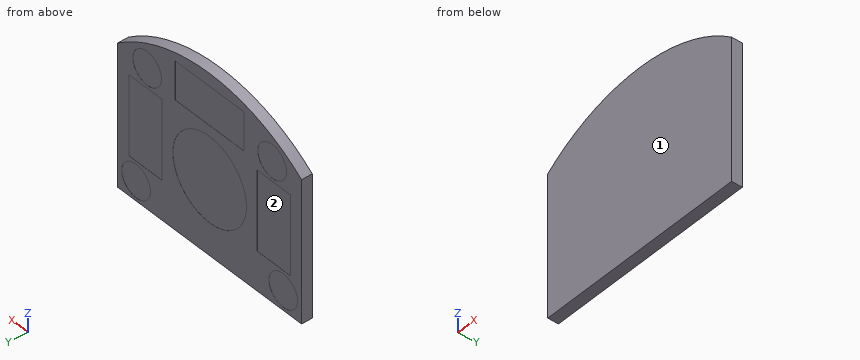
from build123d import *

# Parameters (mm, degrees)
BOSS_EXTRUDE1_DEPTH  = 12.7
BOSS_EXTRUDE2_DEPTH  = 11.176
BOSS_EXTRUDE10_DEPTH = 3.175
SKETCH22_W           = 92.185700808
SKETCH22_H           = 89.424577416
CUT_EXTRUDE13_DEPTH  = 26.4
SKETCH26_W           = 63.5
SKETCH26_H           = 12.7
BOSS_EXTRUDE11_DEPTH = 3.175
SKETCH23_R           = 4.953
SKETCH23_R_2         = 12.7
CUT_EXTRUDE14_DEPTH  = 0.0254
SKETCH25_W           = 11.509375
SKETCH25_H           = 23.8125
SKETCH25_W_2         = 23.8125
SKETCH25_H_2         = 11.509375
CUT_EXTRUDE15_DEPTH  = 0.0254
SKETCH27_W           = 63.5
SKETCH27_H           = 12.7
CUT_EXTRUDE16_DEPTH  = 4.175


with BuildPart() as part:
    # Sketch1 → Boss-Extrude1 (new body)
    with BuildSketch(Plane(origin=(0, 0, 0), x_dir=(1, 0, 0), z_dir=(0, 1, 0))):
        with BuildLine():
            Line((-31.75, 0), (31.75, 0))
            Line((31.75, 0), (31.75, -42.418))
            ThreePointArc((31.75, -42.418), (0, -53.56226271), (-31.75, -42.418))
            Line((-31.75, -42.418), (-31.75, 0))
        make_face()
    extrude(amount=BOSS_EXTRUDE1_DEPTH)

    # Sketch2 → Boss-Extrude2 (add)
    with BuildSketch(Plane.ZY.offset(19.558)):
        with BuildLine():
            Line((0, 0), (-12.7, 0))
            ThreePointArc((-12.7, 0), (-21.680256121, 21.680256121), (0, 12.7))
            Line((0, 12.7), (0, 0))
        make_face()
    boss_extrude2 = extrude(amount=-BOSS_EXTRUDE2_DEPTH)

    # Mirror1: Boss-Extrude2 across plane
    add(boss_extrude2.mirror(Plane(origin=(0, 0, 0), x_dir=(0, 0, 1), z_dir=(1, 0, 0))))

    # Sketch20 → Boss-Extrude10 (add)
    with BuildSketch(Plane.XZ):
        with BuildLine():
            Line((-31.75, 42.418), (-31.75, 0))
            Line((-31.75, 0), (-19.558, 0))
            Line((-19.558, 0), (-19.558, -12.7))
            Line((-19.558, -12.7), (-8.382, -12.7))
            Line((-8.382, -12.7), (-8.382, 0))
            Line((-8.382, 0), (8.382, 0))
            Line((8.382, 0), (8.382, -12.7))
            Line((8.382, -12.7), (19.558, -12.7))
            Line((19.558, -12.7), (19.558, 0))
            Line((19.558, 0), (31.75, 0))
            Line((31.75, 0), (31.75, 42.418))
            ThreePointArc((31.75, 42.418), (0, 53.56226271), (-31.75, 42.418))
        make_face()
    extrude(amount=BOSS_EXTRUDE10_DEPTH)

    # Sketch22 → Cut-Extrude13 (cut, through all)
    with BuildSketch(Plane(origin=(0, 0, 0), x_dir=(-1, 0, 0), z_dir=(0, -1, 0))):
        with Locations((-2.135876507, -13.211147217)):
            Rectangle(SKETCH22_W, SKETCH22_H)
    extrude(amount=-CUT_EXTRUDE13_DEPTH, mode=Mode.SUBTRACT)

    # Sketch26 → Boss-Extrude11 (add)
    with BuildSketch(Plane(origin=(0, 0, 0), x_dir=(1, 0, 0), z_dir=(0, 1, 0))):
        with Locations((0, 6.35)):
            Rectangle(SKETCH26_W, SKETCH26_H)
    extrude(amount=-BOSS_EXTRUDE11_DEPTH)

    # Sketch23 → Cut-Extrude14 (cut)
    with BuildSketch(Plane(origin=(0, 0, 0), x_dir=(1, 0, 0), z_dir=(0, 1, 0))):
        with Locations((25.4, -5.842)):
            Circle(SKETCH23_R)
        with Locations((21.59, -41.402)):
            Circle(SKETCH23_R)
        with Locations((-25.4, -5.842)):
            Circle(SKETCH23_R)
        with Locations((-21.59, -41.402)):
            Circle(SKETCH23_R)
        with Locations((0, -22.32026271)):
            Circle(SKETCH23_R_2)
    extrude(amount=-CUT_EXTRUDE14_DEPTH, mode=Mode.SUBTRACT)

    # Sketch25 → Cut-Extrude15 (cut)
    with BuildSketch(Plane(origin=(0, 0, 0), x_dir=(1, 0, 0), z_dir=(0, 1, 0))):
        with Locations((-22.1853125, -23.62201271)):
            Rectangle(SKETCH25_W, SKETCH25_H)
        with Locations((0, -43.99757521)):
            Rectangle(SKETCH25_W_2, SKETCH25_H_2)
        with Locations((22.1853125, -23.62201271)):
            Rectangle(SKETCH25_W, SKETCH25_H)
    extrude(amount=-CUT_EXTRUDE15_DEPTH, mode=Mode.SUBTRACT)

    # Sketch27 → Cut-Extrude16 (cut, through all)
    with BuildSketch(Plane(origin=(0, 0, 0), x_dir=(1, 0, 0), z_dir=(0, 1, 0))):
        with Locations((0, 6.35)):
            Rectangle(SKETCH27_W, SKETCH27_H)
    extrude(amount=-CUT_EXTRUDE16_DEPTH, mode=Mode.SUBTRACT)


solid = part.part
CAD build for the part. Positions are in the model's coordinates, mm. Face numbers are marked on the shaded views. Coordinates: 2 decimals unless noted, no trailing zeros. Order: outer loops, then holes, each group sorted by start corner. A loop starts at its lowest first (then second) coordinate and runs counter-clockwise, first axis right, second up. Notation, with made-up numbers: (43, -0.5) -> (70, -0.5) arc R19 ccw to (70, 4.5) -> close; hole circle Ø9 at (25.25, 25). An arc over 180 degrees is marked (long way). Answer in a Markdown table with one row per item.
1) Band-saw the part on A-A (x = 21.59). List the corners of the cut face in (y, z) (3 decimals), and give its area (3 significant figures).
Check values:
| item | result |
|---|---|
| outline | (-3.175, 0) -> (0, 0) -> (0, 2.677) -> (-0.025, 2.677) -> (-0.025, 9.007) -> (0, 9.007) -> (0, 11.716) -> (-0.025, 11.716) -> (-0.025, 35.528) -> (0, 35.528) -> (0, 36.449) -> (-0.025, 36.449) -> (-0.025, 46.355) -> (0, 46.355) -> (0, 48.746) -> (-3.175, 48.746) -> close |
| area | 154 mm2 |
2) Drill centre lines: line 1 (Y direction, x = 4, z = 49) (3 decimals); line 2 (X direction, y = -2.75, z = 43.5); line 3 (Z direction, x = 5.5, y = -1.65). Where is each one in solid material? Low to high.
Check values:
| item | result |
|---|---|
| line 1 | -3.175 to -0.025 |
| line 2 | -30.35 to 30.35 |
| line 3 | 0 to 53.26 |
3) Band-saw the part on D-D (x = -15.5). List the corners of the cut face in (y, z) (3 decimals), and give its area (3 significant figures).
Check values:
| item | result |
|---|---|
| outline | (-3.175, 0) -> (0, 0) -> (0, 51.14) -> (-3.175, 51.14) -> close |
| area | 162 mm2 |
4) Flat gauge pin, fed straight in: P1, Ø3, axis at x = 24.5, z = 7.5, coming from the +Y side. Where does the tip first touch, or does it go through?
Check values:
| item | result |
|---|---|
| P1 | y = -0.03 |
5) Band-saw the part on C-C (x = -24). List the corners of the cut face in (y, z) (3 decimals).
Check values:
| item | result |
|---|---|
| outline | (-3.175, 0) -> (0, 0) -> (0, 1.091) -> (-0.025, 1.091) -> (-0.025, 10.593) -> (0, 10.593) -> (0, 11.716) -> (-0.025, 11.716) -> (-0.025, 35.528) -> (0, 35.528) -> (0, 37.075) -> (-0.025, 37.075) -> (-0.025, 45.729) -> (0, 45.729) -> (0, 47.535) -> (-3.175, 47.535) -> close |
6) Band-saw the part on B-B (y = -1.15). List the corners of the cut face in (x, z), and give its area (3 significant figures).
Check values:
| item | result |
|---|---|
| outline | (-31.75, 0) -> (31.75, 0) -> (31.75, 42.42) arc R50.8 ccw to (-31.75, 42.42) -> close |
| area | 3,180 mm2 |
7) Mould opens along Y. For the marked faces 1 and 2 say: pulls with the +Y half, pulls with the -Y half, needs draft (parallel to the pull), parting line crosses it, or undercut.
Check values:
| item | result |
|---|---|
| face 1 | pulls with the -Y half |
| face 2 | pulls with the +Y half |
